Geometry check sheet. Reference: the model listing, model coordinates, mm. Face numbers are marked on the shaded views. A direction names the side the tool comes from. Give positions to 0.01 mm unless a question says otherwise; leave off trailing zeros. Write each loop counter-clockwise with the first axis right and the second up, starting at its lowest first coordinate (ties: lowest second). Pieces come first, ordered by that corner, then holes. Notation, with made-up numbers: (87, 21.25) - (142, 21.25) arc R8 ccw to (142, 26.25) - close; hole circle Ø8 at (85.5, 44). An arc over 180 degrees is marked (long way). Use a Markdown table: item, result.
```python
from build123d import *

# Parameters (mm, degrees)
SKETCH1_W           = 45
SKETCH1_H           = 6
SKETCH1_W_2         = 6
BOSS_EXTRUDE1_DEPTH = 4
SKETCH2_R           = 1.6
CUT_EXTRUDE1_DEPTH  = 52.778373864
FILLET2_SIZE        = 6
FILLET3_R           = 2.5


with BuildPart() as part:
    # Sketch1 → Boss-Extrude1 (new body)
    with BuildSketch(Plane.XY):
        with Locations((-22.5, -3)):
            Rectangle(SKETCH1_W, SKETCH1_H)
        Polygon((-45, 0), (-39, 0), (-39, 8), (-45, 8), (-45, 2), align=None)
        with Locations((-48, 5)):
            Rectangle(SKETCH1_W_2, SKETCH1_H)
    extrude(amount=BOSS_EXTRUDE1_DEPTH)

    # Sketch2 → Cut-Extrude1 (cut, through all)
    with BuildSketch(Plane(origin=(0, 0, 0), x_dir=(-1, 0, 0), z_dir=(0, 0, -1))):
        with Locations((3, -3)):
            Circle(SKETCH2_R)
        with Locations((37, -3)):
            Circle(SKETCH2_R)
        with Locations((48, 5)):
            Circle(SKETCH2_R)
    extrude(amount=-CUT_EXTRUDE1_DEPTH, mode=Mode.SUBTRACT)

    # Fillet2
    # a fillet whose section is not a circle: 6 mm, written as the material it takes off along each edge
    with BuildSketch(Plane(origin=(-45, -6, -15), x_dir=(1, 0, 0), z_dir=(0, 0, 1))) as fillet2_piece_1:
        with BuildLine():
            Bezier((FILLET2_SIZE, 0), (0, 0), (0, FILLET2_SIZE), weights=[1, 0.428571429, 1])
            Line((0, FILLET2_SIZE), (0, 0))
            Line((0, 0), (FILLET2_SIZE, 0))
        make_face()
    extrude(amount=34, mode=Mode.SUBTRACT)
    with BuildSketch(Plane(origin=(-39, 8, -15), x_dir=(0, -1, 0), z_dir=(0, 0, 1))) as fillet2_piece_2:
        with BuildLine():
            Bezier((FILLET2_SIZE, 0), (0, 0), (0, -FILLET2_SIZE), weights=[1, 0.428571429, 1])
            Line((0, -FILLET2_SIZE), (0, 0))
            Line((0, 0), (FILLET2_SIZE, 0))
        make_face()
    extrude(amount=34, mode=Mode.SUBTRACT)

    # Fillet3
    fillet3_edges = [part.edges().sort_by_distance(p)[0] for p in [
        (-51, 8, 2),
        (-51, 2, 2),
        (-45, 2, 2),
        (-39, 0, 2),
        (0, 0, 2),
        (0, -6, 2),
    ]]
    fillet(fillet3_edges, radius=FILLET3_R)


solid = part.part
```
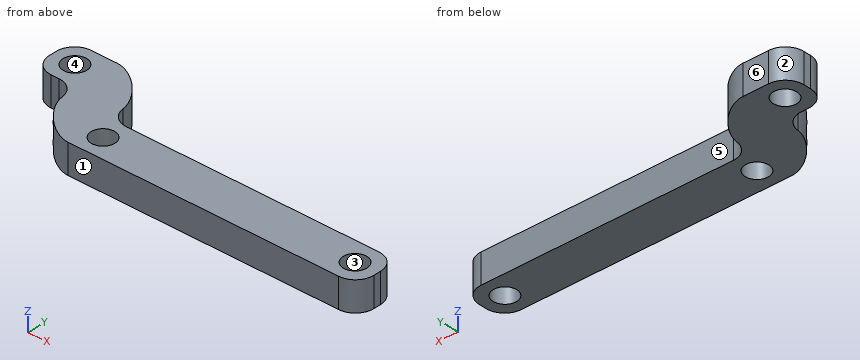
1) Mould release check, pull along X, two halves, no side actions. Record for the marked faces 1, 2, 3 and 4: pulls with the +X half, pulls with the -X half, needs draft (parallel to the pull), parting line crosses it, or undercut.
Working result:
| item | result |
|---|---|
| face 1 | needs draft |
| face 2 | pulls with the -X half |
| face 3 | undercut |
| face 4 | undercut |
2) Section check B-B on z = 1.9. Count the separate pieces of the cut face and the enclosed holes in it, then the cut area to 3 significant figures.
Working result:
| item | result |
|---|---|
| separate pieces | 1 |
| enclosed holes | 3 |
| area | 307 mm² |
3) Material ranges on L1, parallel to Y at x = -48, z = 1.15; L2, parallel to X at y = -2, z = 1.3; L3, parallel to Y at x = -28, z = 3.15, recorded low to high. Write a range as from..to.
Working result:
| item | result |
|---|---|
| L1 | y = 2..3.4, 6.6..8 |
| L2 | x = -44.37..-38.25, -35.75..-4.25, -1.75..-0.05 |
| L3 | y = -6..0 |
4) Section check A-A on x = -3. Record the boundary of the cut face in (y, z), then the cut area to 3 significant figures.
Working result:
| item | result |
|---|---|
| outline | (-6, 0) - (-4.6, 0) - (-4.6, 4) - (-6, 4) - close; (-1.4, 0) - (0, 0) - (0, 4) - (-1.4, 4) - close |
| area | 11.2 mm² |
5) Set-up check for the marked faces 5 and 6: record each of +Z, -Z, +X, -X, +Y, -Y from which the full face is reachable in a straight line by a thin tool's end or side.
Working result:
| item | result |
|---|---|
| face 5 | +Z, -Z, +X, +Y |
| face 6 | +Z, -Z, +X, -X, +Y |
6) Depth check by flat-ended pin: P1, Ø1.1, axis at x = -48, z = 3, coming from the -Y side; P2, Ø1, axis at x = -43, z = 0.5, coming from the -Y side. Enter the tip coordinate at first touch or a pass-through.
Working result:
| item | result |
|---|---|
| P1 | stops at y = 2 |
| P2 | stops at y = -4.28 |
